Solid Edge part; units mm, degrees
sketch "Sketch1" plane through (0, 0, 0) normal (0, -1, 0) x (1, 0, 0)
  line L0 (-45, -45) -> (-37, -45)
  line L1 (-37, -42) -> (-37, -45)
  line L2 (-19.6716, -22.5) -> (-37.3454, -40.1738)
  line L3 (-19.6716, -22.5) -> (19.6716, -22.5)
  line L4 (37.3454, -40.1738) -> (19.6716, -22.5)
  arc A0 (37, -42) -> (37.3454, -40.1738) centre (42, -42) cw
  line L5 (37, -42) -> (37, -45)
  line L6 (37, -45) -> (45, -45)
  line L7 (45, -45) -> (45, -37)
  line L8 (42, -37) -> (45, -37)
  line L9 (25.3284, -22.5) -> (40.1738, -37.3454)
  line L10 (25.3284, -22.5) -> (37.4174, -22.5)
  arc A1 (42, -25.5) -> (37.4174, -22.5) centre (42, -20.5) cw
  line L11 (42, -25.5) -> (45, -25.5)
  line L12 (45, -25.5) -> (45, -15.5)
  line L13 (42, -15.5) -> (45, -15.5)
  line L14 (37.4174, -18.5) -> (21.3284, -18.5)
  line L15 (2.8284, 0) -> (21.3284, -18.5)
  line L16 (21.3284, 18.5) -> (2.8284, 0)
  line L17 (21.3284, 18.5) -> (37.4174, 18.5)
  line L18 (42, 15.5) -> (45, 15.5)
  line L19 (45, 15.5) -> (45, 25.5)
  line L20 (42, 25.5) -> (45, 25.5)
  arc A2 (37.4174, 22.5) -> (42, 25.5) centre (42, 20.5) cw
  line L21 (37.4174, 22.5) -> (25.3284, 22.5)
  line L22 (40.1738, 37.3454) -> (25.3284, 22.5)
  line L23 (42, 37) -> (45, 37)
  line L24 (45, 37) -> (45, 45)
  line L25 (45, 45) -> (37, 45)
  line L26 (37, 42) -> (37, 45)
  arc A3 (37.3454, 40.1738) -> (37, 42) centre (42, 42) cw
  line L27 (19.6716, 22.5) -> (37.3454, 40.1738)
  line L28 (19.6716, 22.5) -> (-19.6716, 22.5)
  line L29 (-37.3454, 40.1738) -> (-19.6716, 22.5)
  line L30 (-37, 42) -> (-37, 45)
  line L31 (-37, 45) -> (-45, 45)
  line L32 (-45, 45) -> (-45, 37)
  line L33 (-42, 37) -> (-45, 37)
  arc A4 (-40.1738, 37.3454) -> (-42, 37) centre (-42, 42) cw
  line L34 (-25.3284, 22.5) -> (-40.1738, 37.3454)
  line L35 (-25.3284, 22.5) -> (-37.4174, 22.5)
  arc A5 (-42, 25.5) -> (-37.4174, 22.5) centre (-42, 20.5) cw
  line L36 (-42, 25.5) -> (-45, 25.5)
  line L37 (-45, 25.5) -> (-45, 15.5)
  line L38 (-42, 15.5) -> (-45, 15.5)
  line L39 (-37.4174, 18.5) -> (-21.3284, 18.5)
  line L40 (-2.8284, 0) -> (-21.3284, 18.5)
  line L41 (-21.3284, -18.5) -> (-2.8284, 0)
  line L42 (-21.3284, -18.5) -> (-37.4174, -18.5)
  arc A6 (-42, -15.5) -> (-37.4174, -18.5) centre (-42, -20.5) cw
  line L43 (-42, -15.5) -> (-45, -15.5)
  line L44 (-45, -15.5) -> (-45, -25.5)
  line L45 (-42, -25.5) -> (-45, -25.5)
  line L46 (-37.4174, -22.5) -> (-25.3284, -22.5)
  line L47 (-40.1738, -37.3454) -> (-25.3284, -22.5)
  arc A7 (-42, -37) -> (-40.1738, -37.3454) centre (-42, -42) cw
  line L48 (-42, -37) -> (-45, -37)
  line L49 (-45, -37) -> (-45, -45)
  arc A8 (-37, -42) -> (-37.3454, -40.1738) centre (-42, -42) ccw
  arc A9 (42, -37) -> (40.1738, -37.3454) centre (42, -42) ccw
  arc A10 (42, -15.5) -> (37.4174, -18.5) centre (42, -20.5) ccw
  arc A11 (37.4174, 18.5) -> (42, 15.5) centre (42, 20.5) ccw
  arc A12 (40.1738, 37.3454) -> (42, 37) centre (42, 42) ccw
  arc A13 (-37.3454, 40.1738) -> (-37, 42) centre (-42, 42) ccw
  arc A14 (-42, 15.5) -> (-37.4174, 18.5) centre (-42, 20.5) ccw
  arc A15 (-42, -25.5) -> (-37.4174, -22.5) centre (-42, -20.5) ccw
  circle A16 centre (-42, -42) radius 1.6
  circle A17 centre (42, -42) radius 1.6
  circle A18 centre (42, -20.5) radius 1.6
  circle A19 centre (-42, -20.5) radius 1.6
  circle A20 centre (-42, 20.5) radius 1.6
  circle A21 centre (-42, 42) radius 1.6
  circle A22 centre (42, 42) radius 1.6
  circle A23 centre (42, 20.5) radius 1.6
  line L50 (-15.6716, 18.5) -> (15.6716, 18.5)
  line L51 (0, 2.8284) -> (15.6716, 18.5)
  line L52 (-15.6716, 18.5) -> (0, 2.8284)
  line L53 (15.6716, -18.5) -> (-15.6716, -18.5)
  line L54 (0, -2.8284) -> (-15.6716, -18.5)
  line L55 (15.6716, -18.5) -> (0, -2.8284)
  dimension "D1" = 42
extrude "Protrusion1" add sketch "Sketch1" against normal blind 3
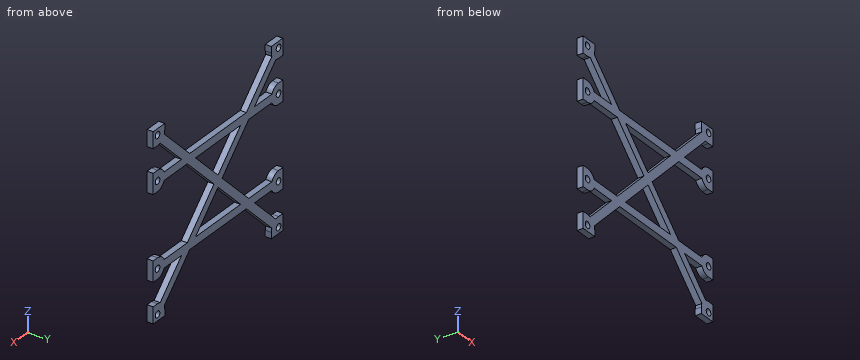
Geometry check sheet. Reference: the model listing, model coordinates, mm. Round coordinates to 2 decimals unless told otherwise and drop trailing zeros. Loops run counter-clockwise (first coordinate to the right, second up) from the corner with the lowest first, then second, coordinate; pieces in that order, holes last. Notation, with made-up numbers: (17, 21.5) - (23, 21.5) arc R11 ccw to (23, 31.5) - close; hole circle Ø11 at (13.5, 20.25). An arc over 180 degrees is marked (long way). One line per question, with ' | ' between items. Start each with the question number.
1. Cross-section at C-C on z = -11.5. Record the cut outline in (x, y), then the cut area to 3 significant figures.
2. Cross-section at B-B on x = 28. Record the cut outline in (y, z).
3. Cross-section at D-D on y = 1.2. State how many separate pieces and enclosed holes the cut face has, then the cut area to 3 significant figures.
4. Cross-section at A-A on z = -20.5. Record the cut outline in (x, y).
5. Scan lines: line 1 (Z direction, x = -32, y = 2.4); line 2 (X direction, y = 1.2, z = 9); line 3 (Z direction, x = -33, y = 1.9). Record each from-to range of solid material in increasing order. Write a range as [from, to].
6. Depth check by flat-ended pin: pin 1 (1 mm diameter, centred on x = 16, y = 0.5, fed in from +Z); pin 2 (2.5 mm diameter, centred on x = -42, z = -42, fed in from +Y); pin 3 (1.5 mm diameter, centred on x = 35.5, y = 2, fed in from -Z); pin 4 (1.5 mm diameter, centred on x = 30.5, y = 1, fed in from +Z). Enter the tip coordinate at first touch or a pass-through.
Taken from the geometry:
1) outline: (-14.33, 0) - (-8.67, 0) - (-8.67, 3) - (-14.33, 3) - close; (8.67, 0) - (14.33, 0) - (14.33, 3) - (8.67, 3) - close | area: 33.9 mm²
2) outline: (0, -30.83) - (3, -30.83) - (3, -25.17) - (0, -25.17) - close; (0, -22.5) - (3, -22.5) - (3, -18.5) - (0, -18.5) - close; (0, 18.5) - (3, 18.5) - (3, 22.5) - (0, 22.5) - close; (0, 25.17) - (3, 25.17) - (3, 30.83) - (0, 30.83) - close
3) separate pieces: 1 | enclosed holes: 10 | area: 1,810 mm²
4) outline: (-45, 0) - (-43.6, 0) - (-43.6, 3) - (-45, 3) - close; (-40.4, 0) - (40.4, 0) - (40.4, 3) - (-40.4, 3) - close; (43.6, 0) - (45, 0) - (45, 3) - (43.6, 3) - close
5) line 1: [-34.83, -29.17], [-22.5, -18.5], [18.5, 22.5], [29.17, 34.83] | line 2: [-11.83, -6.17], [6.17, 11.83] | line 3: [-35.83, -30.17], [-22.5, -18.5], [18.5, 22.5], [30.17, 35.83]
6) pin 1: z = 22.5 | pin 2: through | pin 3: z = -39.08 | pin 4: z = 34.08
